```python
from build123d import *

# Parameters (mm, degrees)
F0_W     = 1024.064392
F0_H     = 524.694004
F1_DEPTH = 21.336
F2_R     = 7.883837
F3_DEPTH = 50.8
F4_R     = 7.571869
F5_DEPTH = 50.8
F6_R     = 7.368514
F7_DEPTH = 50.8
F8_R     = 8.112976
F9_DEPTH = 50.8


with BuildPart() as f1:
    # F0 (on Top) → F1 (new body)
    with BuildSketch(Plane.XY):
        with Locations((373.085335, 229.552608)):
            Rectangle(F0_W, F0_H)
    extrude(amount=-F1_DEPTH)

    # F2 (on face) → F3 (join)
    with BuildSketch(Plane(origin=(0, 0, -21.336), x_dir=(1, 0, 0), z_dir=(0, 0, -1))):
        with Locations((-117.818758, 14.959664)):
            Circle(F2_R)
    extrude(amount=F3_DEPTH)

    # F4 (on face) → F5 (join)
    with BuildSketch(Plane(origin=(0, 0, -21.336), x_dir=(1, 0, 0), z_dir=(0, 0, -1))):
        with Locations((-120.250419, -105.692685)):
            Circle(F4_R)
    extrude(amount=F5_DEPTH)

    # F6 (on face) → F7 (join)
    with BuildSketch(Plane(origin=(0, 0, -21.336), x_dir=(1, 0, 0), z_dir=(0, 0, -1))):
        with Locations((111.060277, -108.45048)):
            Circle(F6_R)
    extrude(amount=F7_DEPTH)

    # F8 (on face) → F9 (join)
    with BuildSketch(Plane(origin=(0, 0, -21.336), x_dir=(1, 0, 0), z_dir=(0, 0, -1))):
        with Locations((112.673059, 16.722616)):
            Circle(F8_R)
    extrude(amount=F9_DEPTH)


solid = f1.part
```
Geometry: final body of the model. Coordinates: model frame, mm. Give positions to 0.01 mm unless a question says otherwise; leave off trailing zeros. Write each loop counter-clockwise with the first axis right and the second up, starting at its lowest first coordinate (ties: lowest second). Pieces come first, ordered by that corner, then holes.
1. Section query A-A, the plane y = 128. Return loops of the section in (x, z).
2. Line query: probe 1 along Z at (x, y) = (114.5, -1). Output: solid intervals per line, ascending.
3. Pin query (flat end, axial travel): P1, Ø3, axis at x = 554, y = 432.5, coming from the -Z side. Return the tip coordinate at first contact, or that it passes through.
4. Section query B-B, the plane x = 451. Return loops of the section in (y, z), then the cut area to 3 significant figures.
5. Section query C-C, the plane z = -31. Return loops of the section in (x, y), then the cut area to 3 significant figures.
Computed:
1. outline: (-138.95, -21.34) - (885.12, -21.34) - (885.12, 0) - (-138.95, 0) - close
2. probe 1: z = -21.34 to 0
3. P1: stops at z = -21.34
4. outline: (-32.79, -21.34) - (491.9, -21.34) - (491.9, 0) - (-32.79, 0) - close
4. area: 11,200 mm2
5. outline: circle Ø15.14 at (-120.25, 105.69); circle Ø15.77 at (-117.82, -14.96); circle Ø14.74 at (111.06, 108.45); circle Ø16.23 at (112.67, -16.72)
5. area: 753 mm2
